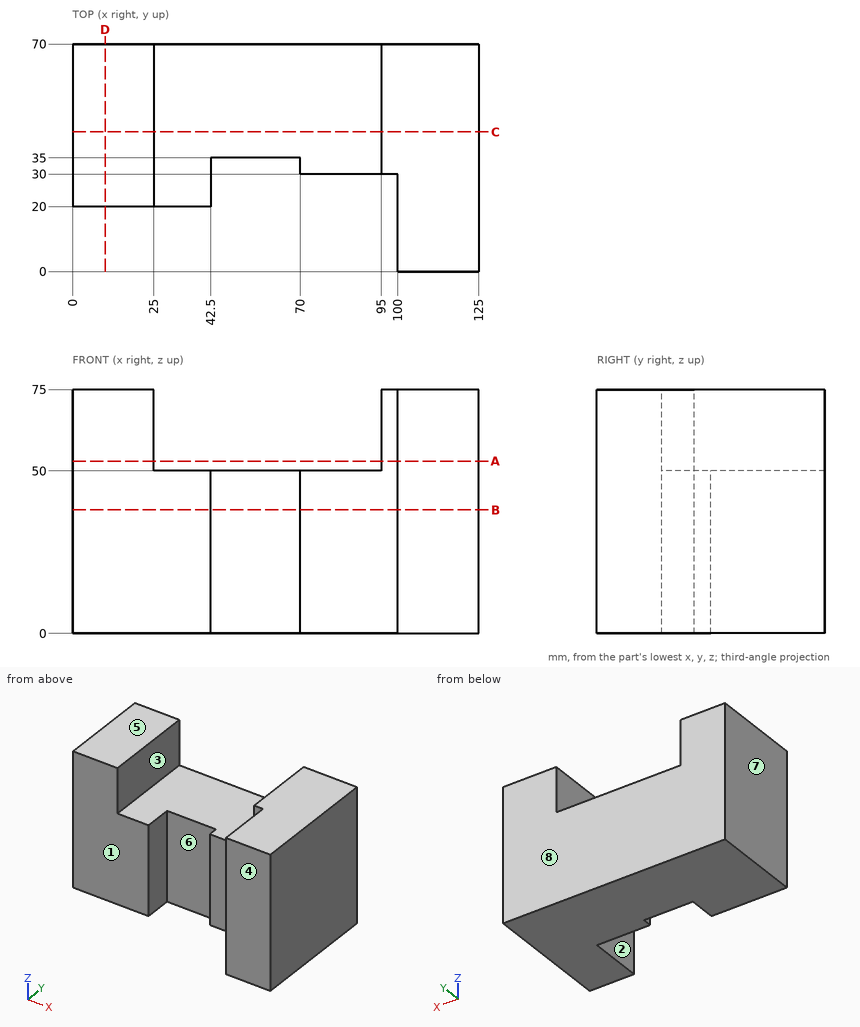
Input: dimensioned drawing with shaded views. Units: mm. Origin: part minimum x, y, z. A direction names the side the tool comes from. Give positions to 0.01 mm unless a question says otherwise; leave off trailing zeros. Write each loop counter-clockwise with the first axis right and the second up, starting at its lowest first coordinate (ties: lowest second). Pieces come first, ordered by that corner, then holes. Notation, with made-up numbers: M 29,-23 L 68,-23 A25 ccw 68,-9 Z; hole C 18.25,11.25 d5. An arc over 180 degrees is marked long. Write item = value, one per line. Start each with the question number.
1) First-contact query: pin 1 Ø14 at (x, z) = (54, 21) entering from -Y; pin 2 Ø1.5 at (x, z) = (20.5, 36) entering from -Y; pin 3 Ø4 at (x, y) = (79, 39) entering from +Z. Flat tips, straight axial feed; report the tip coordinate or a pass-through.
2) Cut plane D-D on x = 10. Return the cut outline in (y, z), then the cut area to 3 significant figures.
3) Cut plane A-A on z = 53. Return the cut outline in (x, y), then the cut area to 3 significant figures.
4) Draft query along X for the marked faces 6, 7 and 8. Return one class per face: +X half, -X half, draft (parallel to the pull), parting line (faces both ways), or undercut.
5) Reachability of the marked faces 1, 2, 3, 4 and 5 from +Z, -Z, +X, -X, +Y, -Y: full face, straight path, thin tool, end or side. Return the list, or none.
6) Cut plane B-B on z = 38. Return the cut outline in (x, y).
7) Material intervals for line 1 along X through (y, z) = (35, 61); line 2 along X through (y, z) = (23, 69); line 3 along Z through (x, y) = (59.5, 37), sorted ascending. Write a range as [from, to].
8) Cut plane C-C on y = 43. Return the cut outline in (x, z).
Solved:
q1.pin_1 = 35
q1.pin_2 = 20
q1.pin_3 = 50
q2.outline = M 20,0 L 70,0 L 70,75 L 20,75 Z
q2.area = 3,750 mm2
q3.outline = M 0,20 L 25,20 L 25,70 L 0,70 Z; M 95,30 L 100,30 L 100,0 L 125,0 L 125,70 L 95,70 Z
q3.area = 3,200 mm2
q4.face_6 = undercut
q4.face_7 = -X half
q4.face_8 = draft
q5.face_1 = +Z, -Z, -X, -Y
q5.face_2 = +Z, -Z, -Y
q5.face_3 = +Z, +Y, -Y
q5.face_4 = +Z, -Z, +X, -X, -Y
q5.face_5 = +Z, +X, -X, +Y, -Y
q6.outline = M 0,20 L 42.5,20 L 42.5,35 L 70,35 L 70,30 L 100,30 L 100,0 L 125,0 L 125,70 L 0,70 Z
q7.line_1 = [0, 25], [95, 125]
q7.line_2 = [0, 25], [100, 125]
q7.line_3 = [0, 50]
q8.outline = M 0,0 L 125,0 L 125,75 L 95,75 L 95,50 L 25,50 L 25,75 L 0,75 Z
